Answer from the drawing. Dimensions are ordinates in mm from the lowest x, y and z of the part. A direction names the side the tool comes from. Round coordinates to 2 decimals unless told otherwise and drop trailing zeros. Loops run counter-clockwise (first coordinate to the right, second up) from the corner with the lowest first, then second, coordinate; pieces in that order, holes last. Notation, with made-up numbers: M 82.25,-6.5 L 121.25,-6.5 A12 ccw 121.25,0.5 Z; hole C 48,84 d9. An arc over 180 degrees is marked long. Answer as a JSON object with one key per item and string values.
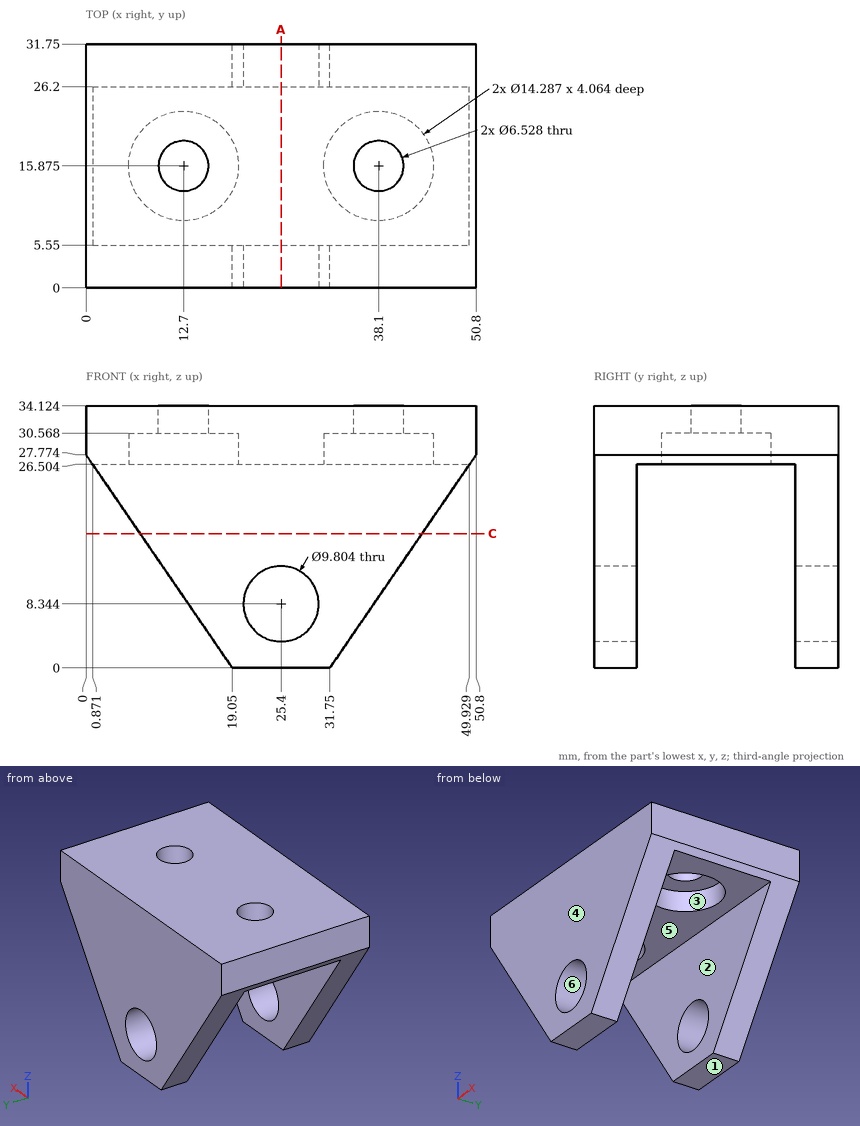
Item 1: Straight lines are drawn through the part: line 1 (Y direction, x = 47, z = 23.5); line 2 (X direction, y = 19.5, z = 30.5) (1 decimal); line 3 (Z direction, x = 35, y = 22.5) (1 decimal). For each, find the intervals that lie inside material, in ascending order.
Values follow:
{"line 1": "0 to 5.55, 26.2 to 31.75", "line 2": "0 to 6.5, 18.9 to 31.9, 44.3 to 50.8", "line 3": "26.5 to 34.1"}
Item 2: The part is cut by section A-A (x = 25.4). Give the number of separate pieces and of enclosed holes in the cut face, then the cut area to 3 significant figures.
Values follow:
{"separate pieces": "3", "enclosed holes": "0", "area": "427 mm^2"}
Item 3: Which of the six approach directions +Z, -Z, +X, -X, +Y, -Y give full straight-line access (tool end or side, diameter ignored) to the marked faces 1, 2 and 3?
Values follow:
{"face 1": "-Z, +X, -X, +Y, -Y", "face 2": "-Z, +X, -X", "face 3": "-Z"}
Item 4: Determine the mould class of the marked faces 4, 5 and 6 for opening direction Y: released by +Y, released by -Y, zero draft, split by the parting line, or undercut.
Values follow:
{"face 4": "released by -Y", "face 5": "undercut", "face 6": "zero draft"}
Item 5: The part is cut by section C-C (z = 17.5). Give the vertices of the cut face in (x, y).
Values follow:
{"outline": "M 7.05,0 L 43.75,0 L 43.75,5.55 L 7.05,5.55 Z; M 7.05,26.2 L 43.75,26.2 L 43.75,31.75 L 7.05,31.75 Z"}
Item 6: Flat-ended cylindrical pins translate along their axes: P1, Ø12, axis at y = 27.5, z = 16.5, coming from the +X side; P2, Ø4, axis at x = 44, y = 13.5, coming from the -Z side; P3, Ø8, axis at y = 10, z = 9.5, coming from the -X side; P4, Ø6, axis at y = 27.5, z = 10, coming from the +X side. Find the tip coordinate at first contact, or state that the pin passes through.
Values follow:
{"P1": "x = 47.18", "P2": "z = 26.5", "P3": "through", "P4": "x = 40.67"}
